Part model, mm, in its own coordinate system. A direction names the side the tool comes from. Coordinates: 2 decimals unless noted, no trailing zeros. Write each loop counter-clockwise with the first axis right and the second up, starting at its lowest first coordinate (ties: lowest second). Pieces come first, ordered by that corner, then holes. Notation, with made-up numbers: (19.25, -33.75) -> (64.25, -33.75) arc R32 ccw to (64.25, 4.25) -> close; hole circle Ø10 at (70.5, 18.25). An arc over 180 degrees is marked (long way). Write item = value, one per line.
Autodesk Inventor part; units mm, degrees
ref_plane "YZ Plane" through (0, 0, 0) normal (1, 0, 0) x (0, 1, 0)
ref_plane "XZ Plane" through (0, 0, 0) normal (0, 1, 0) x (-1, 0, 0)
ref_plane "XY Plane" through (0, 0, 0) normal (0, 0, 1) x (1, 0, 0)
sketch "Sketch1" plane through (0, 0, 0) normal (0, 0, 1) x (1, 0, 0)
  line L0 (0, 0) -> (25.4, 0)
  line L1 (28.575, 3.175) -> (28.575, 28.575)
  line L2 (25.4, 31.75) -> (0, 31.75)
  line L3 (0, 31.75) -> (0, 28.575)
  line L4 (0, 28.575) -> (25.4, 28.575)
  line L5 (25.4, 28.575) -> (25.4, 3.175)
  line L6 (25.4, 3.175) -> (0, 3.175)
  line L7 (0, 3.175) -> (0, 0)
  arc A0 (28.575, 28.575) -> (25.4, 31.75) centre (25.4, 28.575) ccw
  arc A1 (25.4, 0) -> (28.575, 3.175) centre (25.4, 3.175) ccw
  point P0 (28.575, 0)
  point P1 (28.575, 31.75)
  dimension "d0" = 28.575
  dimension "d1" = 31.75
  dimension "d2" = 3.175
  dimension "d3" = 25.4
  dimension "d4" = 25.4
  dimension "d5" = 3.175
extrude "Extrusion1" add sketch "Sketch1" along normal blind 711.2
sketch "Sketch2" plane through (0, 31.75, 0) normal (0, 1, 0) x (1, 0, 0)
  line L0 (25.4, 0) -> (28.575, 0)
  line L1 (25.4, 0) -> (28.575, 0)
  line L2 (28.575, 0) -> (0, -28.575)
  line L3 (0, 0) -> (0, -711.2)
  line L4 (0, -28.575) -> (0, 0)
  line L5 (0, 0) -> (28.575, 0)
  dimension "d8" = 45
extrude "Extrusion2" cut sketch "Sketch2" against normal blind 711.2
sketch "Sketch3" plane through (0, 31.75, 711.2) normal (0, 1, 0) x (1, 0, 0)
  line L0 (0, 0) -> (25.4, 0)
  line L1 (25.4, 0) -> (28.575, 0)
  line L2 (25.4, 0) -> (28.575, 0)
  line L3 (28.575, 0) -> (0, 28.575)
  line L4 (0, 682.625) -> (0, 0)
  line L5 (0, 28.575) -> (0, 0)
  line L6 (0, 0) -> (28.575, 0)
  point P0 (0, 711.2)
  dimension "d11" = 45
extrude "Extrusion3" cut sketch "Sketch3" against normal blind 711.2
properties part number "Chasis 28 piece"
Q1. Saw through at C-C on y = 11.5. Give the cut face in (x, z) (3 decimals), and give its area (3 significant figures).
Model answer:
outline = (25.4, 3.175) -> (28.575, 0) -> (28.575, 711.2) -> (25.4, 708.025) -> close
area = 2,250 mm²
Q2. Saw through at A-A on z = 439.5. Give the cut face in (x, y) (3 decimals).
Model answer:
outline = (0, 0) -> (25.4, 0) arc R3.175 ccw to (28.575, 3.175) -> (28.575, 28.575) arc R3.175 ccw to (25.4, 31.75) -> (0, 31.75) -> (0, 28.575) -> (25.4, 28.575) -> (25.4, 3.175) -> (0, 3.175) -> close
Q3. Which spindle directions (+Z, -Z, +X, -X, +Y, -Y) get a long thin tool onto all of the face, cutting with end or side? Do faces 4 (the face through (13, 3.175, 351)), 5 (the face through (25.996, 14.773, 708.621)). Say none if no direction does.
Model answer:
face_4 = +Z, -Z, -X
face_5 = +Z, -X, +Y, -Y
Q4. Saw through at B-B on x = 18.5. Give the cut face in (y, z) (3 decimals), and give its area (3 significant figures).
Model answer:
outline = (0, 10.075) -> (3.175, 10.075) -> (3.175, 701.125) -> (0, 701.125) -> close; (28.575, 10.075) -> (31.75, 10.075) -> (31.75, 701.125) -> (28.575, 701.125) -> close
area = 4,390 mm²
Q5. Mould opens along Y. For faces 1 (the face through (13, 0, 351)), 2 (the face through (13, 28.575, 351)), 3 (the face through (25.996, 14.773, 2.579)) say: released by +Y, released by -Y, zero draft, split by the parting line, or undercut.
Model answer:
face_1 = released by -Y
face_2 = undercut
face_3 = zero draft
Q6. Probe line 1 (Y direction, x = 4, z = 605) (3 decimals); line 2 (X direction, y = 4.5, z = 192) (3 decimals); line 3 (Z direction, x = 1.5, y = 3) (3 decimals). List the from-to ranges inside material, lowest first. Write a range as from..to.
Model answer:
line_1 = 0..3.175, 28.575..31.75
line_2 = 25.4..28.575
line_3 = 27.075..684.125
Q7. Pin check, flat tip, straight feed: pin 1 (2 mm diameter, centred on y = 6.5, z = 264, fed in from -X). Stop position of the tip, or through.
Model answer:
pin_1 = 25.4
